For this review, take the finished solid that the model builds, in its own axes (mm). Coordinates: 2 decimals unless noted, no trailing zeros. Loops run counter-clockwise (first coordinate to the right, second up) from the corner with the lowest first, then second, coordinate; pieces in that order, holes last. Notation, with made-up numbers: (39.5, 33.5) -> (79.5, 33.5) arc R34 cw to (79.5, 65.5) -> close; hole circle Ø1 at (82, 32.25). An arc over 180 degrees is marked (long way). One line per item, written item: value.
Autodesk Inventor part; units mm, degrees
ref_plane "YZ Plane" through (0, 0, 0) normal (1, 0, 0) x (0, 1, 0)
ref_plane "XZ Plane" through (0, 0, 0) normal (0, 1, 0) x (-1, 0, 0)
ref_plane "XY Plane" through (0, 0, 0) normal (0, 0, 1) x (1, 0, 0)
sketch "Náčrt1" plane through (0, 0, 0) normal (0, 0, 1) x (1, 0, 0)
  line L0 (0, 0) -> (11.831, 0)
  line L1 (11.831, 0) -> (26.7952, 6.9779)
  line L2 (26.7952, 6.9779) -> (24.6821, 11.5094)
  line L3 (24.6821, 11.5094) -> (0, 0)
  line L4 (0, 0) -> (26.7952, 0) construction
  line L5 (18.5187, 6.9803) -> (25.316, 10.15) construction
  line L6 (25.316, 10.15) -> (24.2277, 7.1599) construction
  line L7 (24.2277, 7.1599) -> (26.6578, 1.9486) construction
  line L8 (26.6578, 1.9486) -> (23.9388, 0.6808) construction
  line L9 (23.9388, 0.6808) -> (21.5088, 5.892) construction
  line L10 (21.5088, 5.892) -> (18.5187, 6.9803) construction
  line L11 (23.7275, 1.1339) -> (22.3681, 0.5) construction
  line L12 (26.4465, 2.4018) -> (27.8059, 3.0357) construction
  line L13 (22.3681, 0.5) -> (21.5228, 2.3126) construction
  line L14 (21.5228, 2.3126) -> (26.9607, 4.8483) construction
  line L15 (26.9607, 4.8483) -> (27.8059, 3.0357) construction
  line L16 (50, 0) -> (58.2817, 0)
  line L17 (58.2817, 0) -> (75.5016, 8.0297)
  line L18 (75.5016, 8.0297) -> (74.0224, 11.2018)
  line L19 (74.0224, 11.2018) -> (50, 0)
  line L20 (50, 0) -> (75.5016, 0) construction
  line L21 (69.7022, 8.6356) -> (72.1322, 3.4243) construction
  line L22 (72.1322, 3.4243) -> (71.0439, 0.4342) construction
  line L23 (71.0439, 0.4342) -> (77.8412, 3.6039) construction
  line L24 (77.8412, 3.6039) -> (74.8511, 4.6922) construction
  line L25 (74.8511, 4.6922) -> (72.4211, 9.9034) construction
  line L26 (72.4211, 9.9034) -> (69.7022, 8.6356) construction
  line L27 (21.9174, 8.5652) -> (21.2834, 9.9246) construction
  line L28 (71.0616, 9.2695) -> (70.8503, 9.7227) construction
  dimension "d8" = 5
  dimension "d9" = 25
  dimension "d11" = 8
  dimension "d12" = 3
  dimension "d13" = 45
  dimension "d14" = 7.5
  dimension "d16" = 0
  dimension "d17" = 6
  dimension "d18" = 0.5
  dimension "d19" = 0.5
  dimension "d20" = 2
  dimension "d21" = 27.2337
  dimension "d22" = 3.5
  dimension "d23" = 25
  dimension "d34" = 26.5058
  dimension "d35" = 50
  dimension "d36" = 45
  dimension "d37" = 3
  dimension "d38" = 7.5
  dimension "d39" = 8
  dimension "d42" = 2
  dimension "d44" = 2
  dimension "d59" = 5
  dimension "d63" = 0.5
  dimension "d64" = 19
  dimension "d65" = 0.4342
extrude "Vysunutí1" add sketch "Náčrt1" along normal mid plane 99 contours L19 L18 L17 L16
sketch "Náčrt3" plane through (50, 0, 49.5) normal (-0.4226, 0.9063, 0) x (0.9063, 0.4226, 0)
  line L0 (23.0058, 49.5) -> (23.0058, 82.5) construction
  line L1 (23.0058, 82.5) -> (23.0058, 115.5) construction
  line L2 (0, 99) -> (26.5058, 99)
  line L3 (23.0058, 49.5) -> (23.0058, 16.5) construction
  point P0 (-45.3154, 49.5)
  point P1 (23.0058, 99)
hole "Díra2" at (70.8503, 9.7227, 0) at (70.8503, 9.7227, -33) at (70.8503, 9.7227, 33) direction (0.4226, -0.9063, 0) diameter 3 end through all
thread "Závit1"
thread "Závit2"
thread "Závit3"
properties part number "lowerRamp" material "Ocel, uhlík"
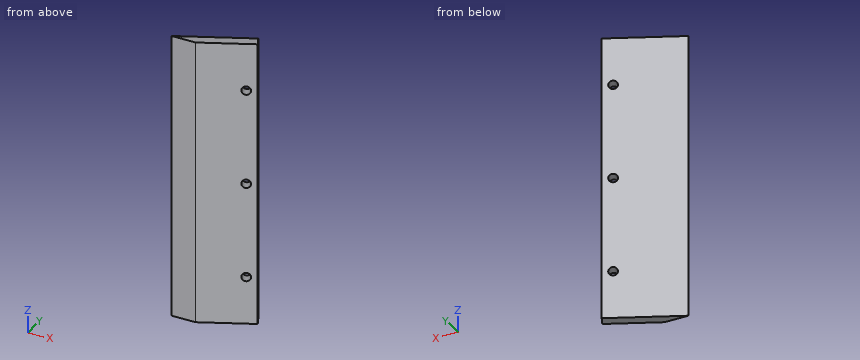
1. To check wall thickness, follow probe 1 along Y at (x, z) = (54, 44); probe 2 along Y at (x, z) = (55, -19.5); probe 3 along X at (y, z) = (4, 17). State the ranges of each line that lie inside material, in increasing order. Write a range as from..to.
Return value:
probe 1: y = 0..1.87
probe 2: y = 0..2.33
probe 3: x = 58.58..66.86
2. Insertion check: pin 1 Ø2 at (x, z) = (70.5, 30.5) entering from -Y; pin 2 Ø2 at (x, z) = (68.5, -6.5) entering from -Y; pin 3 Ø10 at (x, z) = (55, 11.5) entering from +Y. Each pin has a flat end and moves straight along its axis. Give the tip position at first contact, or say it passes through.
Return value:
pin 1: stops at y = 5.23
pin 2: stops at y = 4.3
pin 3: stops at y = 4.66
3. Take a section at B-B, the plane y = 5. Give the boundary of the cut face in (x, z).
Return value:
outline: (60.72, -49.5) -> (69, -49.5) -> (69, 49.5) -> (60.72, 49.5) -> close
4. Take a section at A-A, the plane z = -17.5. Give the boundary of the cut face in (x, y).
Return value:
outline: (50, 0) -> (58.28, 0) -> (75.5, 8.03) -> (74.02, 11.2) -> close
